Here's the drawing with two shaded views (mm, measured from the low corner). I have some questions. A direction names the side the tool comes from. Give positions to 0.01 mm unless a question says otherwise; leave off trailing zeros. Write each loop counter-clockwise with the first axis right and the second up, starting at its lowest first coordinate (ties: lowest second). Pieces come first, ordered by that corner, then holes. Notation, with made-up numbers: M -33,48.5 L -29,48.5 A19 cw -29,70.5 Z; hole C 51.5,45 d1. An arc over 180 degrees is marked long. Answer as a JSON object with one key per item and string values. Group by question number.
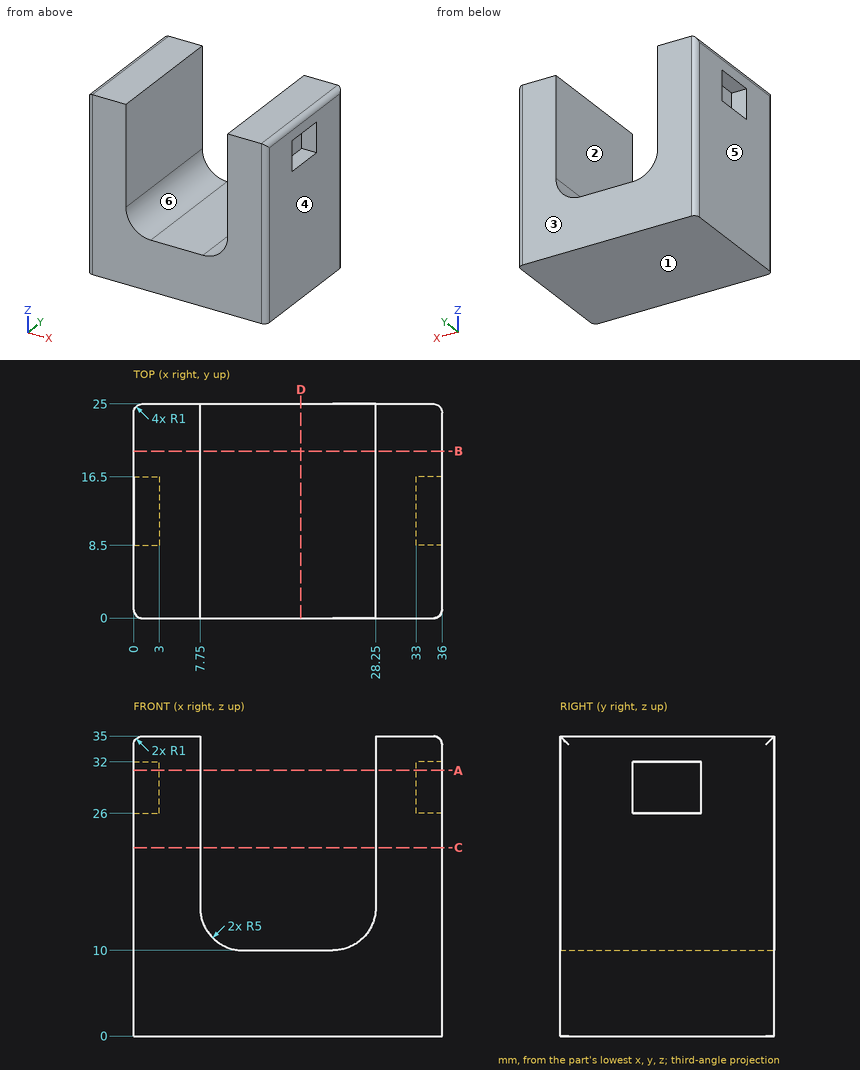
1) If we section it at C-C, the plane z = 22: List the corners of the cut face in (x, y) for me, plus the area to 3 significant figures.
2) If we section it at A-A, the plane z = 31: List the corners of the cut face in (x, y) for me.
3) I'm going to push flat-ended pins straight in: pin 1 (3 mm diameter, centred on x = 17.5, y = 21, fed in from +Z); pin 2 (4 mm diameter, centred on x = 22.5, y = 14, fed in from +Z). Where does each tip first touch, or does it pass through?
4) We'd pull the mould along X, two halves only. Please class the marked faces 3, 4, 5 and 6: released by +X, released by -X, zero draft, split by the parting line, or undercut.
5) If we section it at B-B, the plane y = 19.5: List the corners of the cut face in (x, z) for me, plus the area to 3 significant figures.
6) If we section it at D-D, the plane x = 19.5: List the corners of the cut face in (y, z) for me, plus the area to 3 significant figures.
7) Please list where these lines run through material, in increasing order: line 1 along X through (y, z) = (7.5, 24); line 2 along Y through (x, z) = (34.5, 28); line 3 along Z through (x, y) = (19, 21.25). Write a range as from..to.
8) For the marked faces 1 and 2, which set-ups out of +Z, -Z, +X, -X, +Y, -Y let a thin tool reach every point of the face, with its end or its side?
Taken from the geometry:
{
 "1": {"outline": "M 0,1 A1 ccw 1,0 L 7.75,0 L 7.75,25 L 1,25 A1 ccw 0,24 Z; M 28.25,0 L 35,0 A1 ccw 36,1 L 36,24 A1 ccw 35,25 L 28.25,25 Z", "area": "387 mm²"},
 "2": {"outline": "M 0,1 A1 ccw 1,0 L 7.75,0 L 7.75,25 L 1,25 A1 ccw 0,24 L 0,16.5 L 3,16.5 L 3,8.5 L 0,8.5 Z; M 28.25,0 L 35,0 A1 ccw 36,1 L 36,8.5 L 33,8.5 L 33,16.5 L 36,16.5 L 36,24 A1 ccw 35,25 L 28.25,25 Z"},
 "3": {"pin 1": "z = 10", "pin 2": "z = 10.16"},
 "4": {"face 3": "zero draft", "face 4": "released by +X", "face 5": "released by -X", "face 6": "undercut"},
 "5": {"outline": "M 0,0 L 36,0 L 36,34 A1 ccw 35,35 L 28.25,35 L 28.25,15 A5 cw 23.25,10 L 12.75,10 A5 cw 7.75,15 L 7.75,35 L 1,35 A1 ccw 0,34 Z", "area": "758 mm²"},
 "6": {"outline": "M 0,0 L 25,0 L 25,10 L 0,10 Z", "area": "250 mm²"},
 "7": {"line 1": "0..7.75, 28.25..36", "line 2": "0..8.5, 16.5..25", "line 3": "0..10"},
 "8": {"face 1": "-Z, +X, -X, +Y, -Y", "face 2": "+Z, +Y, -Y"}
}
